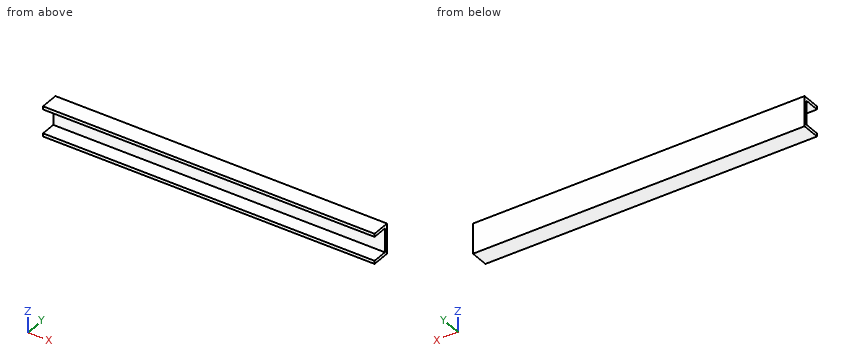
from build123d import *

# Parameters (mm, degrees)
F0_W     = 838.2
F0_H     = 76.2
F1_DEPTH = 7.9375
F2_W     = 838.2
F2_H     = 7.9375
F3_DEPTH = 38.1


with BuildPart() as f1:
    # F0 (on Front) → F1 (new body)
    with BuildSketch(Plane.XZ):
        with Locations((419.1, 38.1)):
            Rectangle(F0_W, F0_H)
    extrude(amount=-F1_DEPTH)

    # F2 (on Front) → F3 (join)
    with BuildSketch(Plane.XZ):
        with Locations((419.1, 72.23125)):
            Rectangle(F2_W, F2_H)
        with Locations((419.1, 3.96875)):
            Rectangle(F2_W, F2_H)
    extrude(amount=F3_DEPTH)


solid = f1.part
Design review of the part built by this model. Coordinates are the model's own, in mm. Round coordinates to 2 decimals unless told otherwise and drop trailing zeros. Write each loop counter-clockwise with the first axis right and the second up, starting at its lowest first coordinate (ties: lowest second). Pieces come first, ordered by that corner, then holes. Notation, with made-up numbers: (16, 61.5) -> (75, 61.5) arc R19 ccw to (75, 85.5) -> close; hole circle Ø7 at (9, 72). An arc over 180 degrees is marked (long way). One line per item, written item: value. Start each with the question number.
Q1. Add section A-A (y = -15). Give the boundary of the cut face in (x, z), then the cut area to 3 significant figures.
Q2. Add section C-C (z = 18.5). Give the boundary of the cut face in (x, y).
Q3. Insertion check: P1, Ø1, axis at x = 186.5, z = 61.5, coming from the -Y side. The pin has a flat end and moves straight along its axis. Give the tip position at first contact, or say it passes through.
Q4. To check wall thickness, follow probe 1 along Z at (x, y) = (103, -19); probe 2 along Y at (x, z) = (292, 22.5). State the ranges of each line that lie inside material, in increasing order.
Q5. Add section B-B (x = 308.5). Give the boundary of the cut face in (y, z), then the cut area to 3 significant figures.
Response:
1. outline: (0, 0) -> (838.2, 0) -> (838.2, 7.94) -> (0, 7.94) -> close; (0, 68.26) -> (838.2, 68.26) -> (838.2, 76.2) -> (0, 76.2) -> close
1. area: 13,300 mm^2
2. outline: (0, 0) -> (838.2, 0) -> (838.2, 7.94) -> (0, 7.94) -> close
3. P1: stops at y = 0
4. probe 1: z = 0 to 7.94, 68.26 to 76.2
4. probe 2: y = 0 to 7.94
5. outline: (-38.1, 0) -> (7.94, 0) -> (7.94, 76.2) -> (-38.1, 76.2) -> (-38.1, 68.26) -> (0, 68.26) -> (0, 7.94) -> (-38.1, 7.94) -> close
5. area: 1,210 mm^2
